from build123d import *

# Parameters (mm, degrees)
SKETCH1_W           = 440
SKETCH1_H           = 1500
BOSS_EXTRUDE1_DEPTH = 80
SKETCH4_W           = 40
SKETCH4_H           = 50
BOSS_EXTRUDE4_DEPTH = 320


with BuildPart() as part:
    # Sketch1 → Boss-Extrude1 (new body)
    with BuildSketch(Plane.XY):
        Rectangle(SKETCH1_W, SKETCH1_H)
    extrude(amount=BOSS_EXTRUDE1_DEPTH)

    # Sketch4 → Boss-Extrude4 (add)
    with BuildSketch(Plane.XY.offset(80)):
        with Locations((-200, 525)):
            Rectangle(SKETCH4_W, SKETCH4_H)
        with Locations((-200, -525)):
            Rectangle(SKETCH4_W, SKETCH4_H)
        with Locations((200, -525)):
            Rectangle(SKETCH4_W, SKETCH4_H)
        with Locations((200, 525)):
            Rectangle(SKETCH4_W, SKETCH4_H)
    extrude(amount=BOSS_EXTRUDE4_DEPTH)


solid = part.part
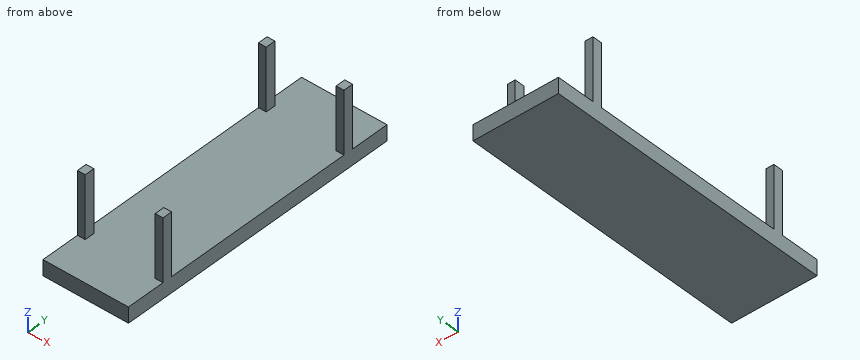
Read the model definition and answer for the solid it produces. Units are mm, in the model's axes. Round coordinates to 2 decimals unless told otherwise and drop trailing zeros. Order: outer loops, then holes, each group sorted by start corner. A loop starts at its lowest first (then second) coordinate and runs counter-clockwise, first axis right, second up. Notation, with made-up numbers: (50.25, 6.5) - (87.25, 6.5) arc R13 cw to (87.25, 24.5) - close; hole circle Ø5 at (43.25, 17.25). An arc over 180 degrees is marked (long way). Use one line per item in the form item = value. Start each with the question number.
(1) The part is cut by section A-A (z = 102). Give the vertices of the cut face in (x, y).
(2) Find the intervals of material crossed by line 1 along X through (y, z) = (535, 374.5); line 2 along Z through (x, y) = (-86.5, 565.5), in increasing order. Write a range as from..to.
(3) Flat-ended cylindrical pins translate along their axes: pin 1 Ø20 at (x, z) = (-194.5, 290.5) entering from +Y; pin 2 Ø12 at (x, z) = (-191.5, 228.5) entering from -Y; pin 3 Ø5 at (x, y) = (-136, 239.5) entering from +Z. Find the tip coordinate at first contact, or state that the pin passes through.
(4) The part is cut by section C-C (y = 520). Give the vertices of the cut face in (x, z).
(5) The part is cut by section B-B (x = 193.5). Give the vertices of the cut face in (y, z).
Checked values:
q1.outline = (-220, -550) - (-180, -550) - (-180, -500) - (-220, -500) - close; (-220, 500) - (-180, 500) - (-180, 550) - (-220, 550) - close; (180, -550) - (220, -550) - (220, -500) - (180, -500) - close; (180, 500) - (220, 500) - (220, 550) - (180, 550) - close
q2.line_1 = -220..-180, 180..220
q2.line_2 = 0..80
q3.pin_1 = 550
q3.pin_2 = -550
q3.pin_3 = 80
q4.outline = (-220, 0) - (220, 0) - (220, 400) - (180, 400) - (180, 80) - (-180, 80) - (-180, 400) - (-220, 400) - close
q5.outline = (-750, 0) - (750, 0) - (750, 80) - (550, 80) - (550, 400) - (500, 400) - (500, 80) - (-500, 80) - (-500, 400) - (-550, 400) - (-550, 80) - (-750, 80) - close
